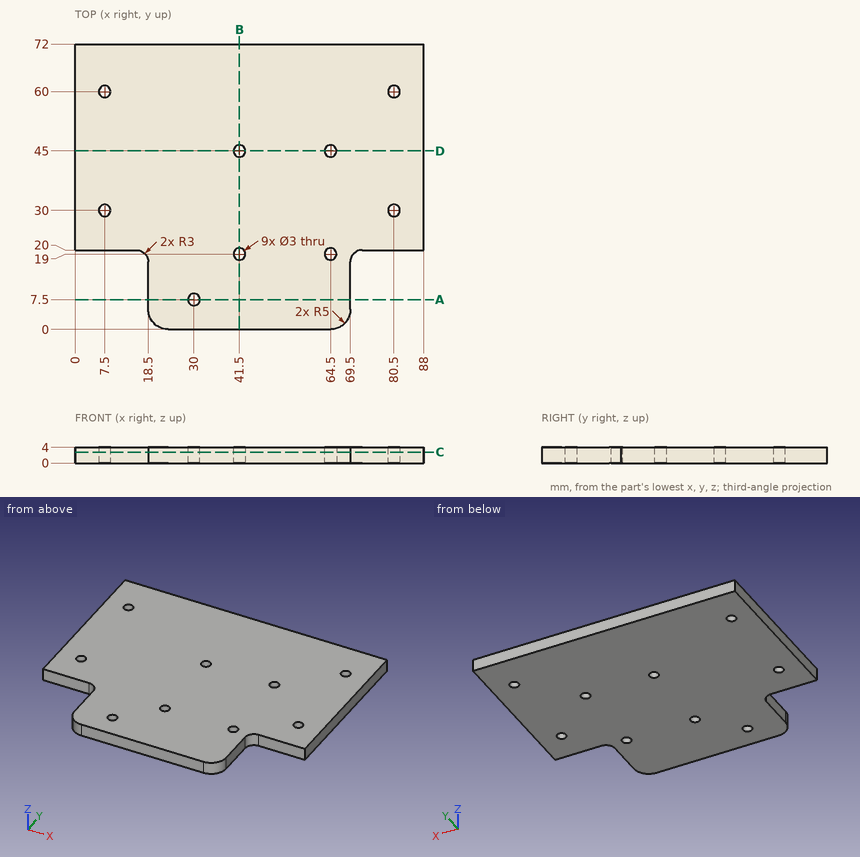
Geometry check sheet. Reference: drawing and pictorial views, mm from the part's lowest x, y, z. Coordinates: 2 decimals unless noted, no trailing zeros. Write each loop counter-clockwise with the first axis right and the second up, starting at its lowest first coordinate (ties: lowest second). Pieces come first, ordered by that corner, then holes. Notation, with made-up numbers: (85, 25) -> (132, 25) arc R27 cw to (132, 41) -> close; hole circle Ø2 at (17.5, 81). An arc over 180 degrees is marked (long way). Use a Markdown table: item, result.
1. Scan lines: line 1 along Y through (x, z) = (80.5, 1.4); line 2 along Y through (x, z) = (30, 2); line 3 along Y through (x, z) = (82.5, 2.3). Record each from-to range of solid material in increasing order.
Reported:
| item | result |
|---|---|
| line 1 | y = 20 to 28.5, 31.5 to 58.5, 61.5 to 72 |
| line 2 | y = 0 to 6, 9 to 72 |
| line 3 | y = 20 to 72 |
2. Sectioned sample at B-B (x = 41.5). Enter the section's corners in (y, z).
Reported:
| item | result |
|---|---|
| outline | (0, 0) -> (17.5, 0) -> (17.5, 4) -> (0, 4) -> close; (20.5, 0) -> (43.5, 0) -> (43.5, 4) -> (20.5, 4) -> close; (46.5, 0) -> (72, 0) -> (72, 4) -> (46.5, 4) -> close |
3. Go/stop test with flat-tipped pins: pin 1 Ø1.2 at (x, z) = (83, 1.5) entering from -Y; pin 2 Ø2.5 at (x, y) = (64.5, 19) entering from -Z; pin 3 Ø1 at (y, z) = (19, 3) entering from +X; pin 4 Ø1.2 at (y, z) = (8.5, 2.5) entering from +X. Record where each tip stops, or that it passes through.
Reported:
| item | result |
|---|---|
| pin 1 | stops at y = 20 |
| pin 2 | passes through |
| pin 3 | stops at x = 70.84 |
| pin 4 | stops at x = 69.5 |
4. Sectioned sample at D-D (y = 45). Enter the section's corners in (x, z), plus the area to 3 significant figures.
Reported:
| item | result |
|---|---|
| outline | (0, 0) -> (40, 0) -> (40, 4) -> (0, 4) -> close; (43, 0) -> (63, 0) -> (63, 4) -> (43, 4) -> close; (66, 0) -> (88, 0) -> (88, 4) -> (66, 4) -> close |
| area | 328 mm2 |
5. Sectioned sample at A-A (y = 7.5). Enter the section's corners in (x, z).
Reported:
| item | result |
|---|---|
| outline | (18.5, 0) -> (28.5, 0) -> (28.5, 4) -> (18.5, 4) -> close; (31.5, 0) -> (69.5, 0) -> (69.5, 4) -> (31.5, 4) -> close |
6. Sectioned sample at C-C (z = 2.75). Give the number of separate pieces and of enclosed holes in the cut face, plus the area to 3 significant figures.
Reported:
| item | result |
|---|---|
| separate pieces | 1 |
| enclosed holes | 9 |
| area | 5,530 mm2 |
